Design review of the part built by this model. Coordinates are the model's own, in mm. A direction names the side the tool comes from. Give positions to 0.01 mm unless a question says otherwise; leave off trailing zeros. Loops run counter-clockwise (first coordinate to the right, second up) from the corner with the lowest first, then second, coordinate; pieces in that order, holes last.
from build123d import *

# Parameters (mm, degrees)
BOSS_EXTRUDE1_DEPTH = 3.175
CUT_EXTRUDE1_REACH  = 71.579
SKETCH2_W           = 5.08
SKETCH2_H           = 6.35


with BuildPart() as part:
    # Sketch1 → Boss-Extrude1 (new body)
    with BuildSketch(Plane.XY):
        Polygon((4.219666631, 0), (-4.219666631, 0), (-40.641770339, -52.016154812), (-34.399831762, -56.386807257), (-3.81, -12.7), (3.81, -12.7), (34.399831762, -56.386807257), (40.641770339, -52.016154812), align=None)
    extrude(amount=BOSS_EXTRUDE1_DEPTH)

    # Sketch2 → Cut-Extrude1 (cut, up to next)
    with BuildSketch(Plane.XY.offset(3.175), mode=Mode.PRIVATE) as cut_extrude1_sk1:
        with Locations((0, -3.175)):
            Rectangle(SKETCH2_W, SKETCH2_H)
    cut_extrude1_tool1 = extrude(cut_extrude1_sk1.sketch, amount=-CUT_EXTRUDE1_REACH, mode=Mode.PRIVATE) & part.part
    add(cut_extrude1_tool1.solids().sort_by_distance((0, -3.175, 3.175))[0], mode=Mode.SUBTRACT)


solid = part.part
Q1. Take a section at C-C (x = -28.5). Give the boundary of the cut face in (y, z) (3 decimals), plus the area to 3 significant figures.
Results:
outline: (-47.961, 0) - (-34.676, 0) - (-34.676, 3.175) - (-47.961, 3.175) - close
area: 42.2 mm2
Q2. Insertion check: pin 1 (1.5 mm diameter, centred on x = -10, z = 0.5, fed in from -Y); pin 2 (1 mm diameter, centred on x = 20, z = 1.5, fed in from +Y); pin 3 (4 mm diameter, centred on x = -13, y = -15, fed in from -Z); pin 4 (1.6 mm diameter, centred on x = 1, z = 2, fed in from -Y). Each pin has a flat end and moves straight along its axis. Give the tip position at first contact, or say it passes through.
Results:
pin 1: stops at y = -22.61
pin 2: stops at y = -21.82
pin 3: stops at z = 0
pin 4: stops at y = -12.7
Q3. Draft analysis for pull direction X (two halves, no side actions). For faces 1 (the face through (22.686, -26.372, 1.565)), 2 (the face through (0, -6.35, 2)), 3 (the face through (12, -24, 0)), 4 (the face through (-22.176, -25.644, 1.565)), state which applies: pulls with the +X half, pulls with the -X half, needs draft (parallel to the pull), parting line crosses it, or undercut.
Results:
face 1: pulls with the +X half
face 2: undercut
face 3: needs draft
face 4: pulls with the -X half
Q4. Take a section at D-D (y = -11). Give the boundary of the cut face in (x, z) (3 decimals).
Results:
outline: (-11.922, 0) - (11.922, 0) - (11.922, 3.175) - (-11.922, 3.175) - close
Q5. Take a section at A-A (z = 0.75). Give the boundary of the cut face in (x, y).
Results:
outline: (-40.64, -52.02) - (-34.4, -56.39) - (-3.81, -12.7) - (3.81, -12.7) - (34.4, -56.39) - (40.64, -52.02) - (4.22, 0) - (2.54, 0) - (2.54, -6.35) - (-2.54, -6.35) - (-2.54, 0) - (-4.22, 0) - close
Q6. Take a section at B-B (y = -44). Give the boundary of the cut face in (x, z) (1 decimal).
Results:
outline: (-35, 0) - (-25.7, 0) - (-25.7, 3.2) - (-35, 3.2) - close; (25.7, 0) - (35, 0) - (35, 3.2) - (25.7, 3.2) - close
Q7. Wall thickness on line 1 (Y direction, x = 3, z = 0.75); line 2 (X direction, y = -39, z = 2.8); line 3 (X direction, y = -49, z = 1.3): over which ranges is each line inside the solid? List them lowest first.
Results:
line 1: y = -12.7 to 0
line 2: x = -31.53 to -22.23, 22.23 to 31.53
line 3: x = -38.53 to -29.23, 29.23 to 38.53
Q8. Tool access review of faces 5 (the face through (2.54, -3, 2)), 6 (the face through (18.891, -34.238, 1.565)), 7 (the face through (-3, 0, 2)): name each direction out of +Z, -Z, +X, -X, +Y, -Y from which nothing blocks a thin tool from reaching the whole face with its end or side.
Results:
face 5: +Z, -Z, +Y
face 6: +Z, -Z, -Y
face 7: +Z, -Z, +X, -X, +Y
